Check sheet for the modelled part. Datum: model origin and axes. Units: mm. A direction names the side the tool comes from. Give positions to 0.01 mm unless a question says otherwise; leave off trailing zeros. Order: outer loops, then holes, each group sorted by start corner. A loop starts at its lowest first (then second) coordinate and runs counter-clockwise, first axis right, second up.
Item 1: Sectioned sample at B-B on x = 162. Record the boundary of the cut face in (y, z).
Item 2: Access from +Z, -Z, +X, -X, +Y, -Y to the whole of each face (thin tool, end or side, straight path). Record for faces 4 (the flat face through (159.24, 186.98, 5.92)), 5 (the flat face through (162.396, 182, 6)).
Item 3: Material ranges on line 1 along X through (y, z) = (183.75, 3.25); line 2 along X through (y, z) = (175.25, 7.75); line 3 along Y through (x, z) = (162.5, 5), recorded low to high.
Item 4: Sectioned sample at C-C on y = 176.5. Record the boundary of the cut face in (x, z).
Item 5: Gauge pin test, flat ends, axial feed: P1, Ø1, axis at y = 185.5, z = 9, coming from the +X side; P2, Ø3.5, axis at y = 177, z = 6.5, coming from the -X side; P3, Ø2, axis at x = 153, z = 6.5, coming from the -Y side. Record the tip position at first contact, or that the pin passes through.
Item 6: Sectioned sample at A-A on y = 168.75. Record the boundary of the cut face in (x, z).
Item 7: Release check for a two-part mould opening along Y. For faces 1 (the flat face through (164, 175.551, 6)), 2 (the cylindrical face through (148.213, 162.985, 5.916)), 3 (the flat face through (158.766, 180, 6)) record: released by +Y, released by -Y, zero draft, split by the parting line, or undercut.
Item 8: Sectioned sample at D-D on x = 152.25. Record the boundary of the cut face in (y, z).
from build123d import *

# Parameters (mm, degrees)
ESQUISSE1_R        = 1.3
BOSS_EXTRU_1_DEPTH = 12


with BuildPart() as part:
    # Esquisse1 → Boss.-Extru.1 (new body)
    with BuildSketch(Plane.XY):
        with BuildLine():
            Line((159.701668195, 188.296706066), (158.766015625, 185.623295296))
            Line((158.766015625, 185.623295296), (158.766015625, 173.839174165))
            add(Edge.make_bspline(
                [(158.766015625, 173.839174165), (158.908011503, 171.16248829), (154.528686771, 169.726069)],
                knots=[0, 0, 0, 1, 1, 1], degree=2))
            Line((154.528686771, 169.726069), (147.466091463, 167.071838941))
            ThreePointArc((147.466091463, 167.071838941), (145.677207205, 163.224776021), (149.524270126, 161.435891763))
            Line((149.524270126, 161.435891763), (162.793418929, 166.356678901))
            ThreePointArc((162.793418929, 166.356678901), (164.222709959, 167.45524387), (164.764329598, 169.17465249))
            Line((164.764329598, 169.17465249), (164.764329598, 175.550568138))
            Line((164.764329598, 175.550568138), (162.39595917, 175.550568138))
            Line((162.39595917, 175.550568138), (162.39595917, 188.296706066))
            Line((162.39595917, 188.296706066), (159.701668195, 188.296706066))
        make_face()
        with Locations((148.495180794, 164.253865352)):
            Circle(ESQUISSE1_R, mode=Mode.SUBTRACT)
        with Locations((161.764329598, 169.17465249)):
            Circle(ESQUISSE1_R, mode=Mode.SUBTRACT)
    extrude(amount=BOSS_EXTRU_1_DEPTH)


solid = part.part
Report:
1. outline: (166.06, 0) - (167.9, 0) - (167.9, 12) - (166.06, 12) - close; (170.45, 0) - (188.3, 0) - (188.3, 12) - (170.45, 12) - close
2. face 4: +Z, -Z, -X, +Y
2. face 5: +Z, -Z, +X, +Y
3. line 1: x = 158.77 to 162.4
3. line 2: x = 158.77 to 164.76
3. line 3: y = 166.25 to 168.1, 170.25 to 175.55
4. outline: (158.77, 0) - (162.4, 0) - (162.4, 12) - (158.77, 12) - close
5. P1: stops at x = 162.4
5. P2: stops at x = 158.77
5. P3: stops at y = 162.35
6. outline: (151.93, 0) - (160.54, 0) - (160.54, 12) - (151.93, 12) - close; (162.99, 0) - (164.73, 0) - (164.73, 12) - (162.99, 12) - close
7. face 1: released by +Y
7. face 2: undercut
7. face 3: zero draft
8. outline: (162.45, 0) - (168.87, 0) - (168.87, 12) - (162.45, 12) - close
